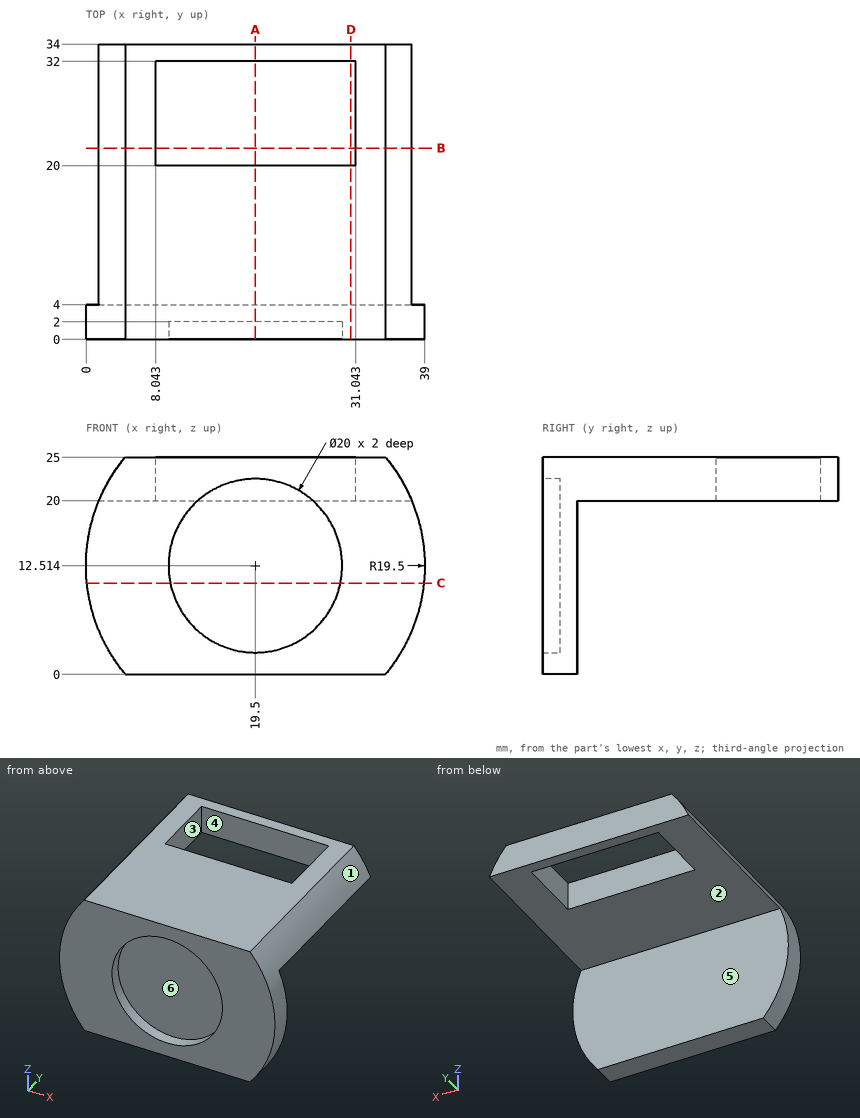
Could you check a few things on this drawing? It's one solid part, dimensions in mm from its lowest x, y, z. A direction names the side the tool comes from. Give positions to 0.01 mm unless a question says otherwise; leave off trailing zeros. Write each loop counter-clockwise with the first axis right and the second up, starting at its lowest first coordinate (ties: lowest second). Pieces come first, ordered by that corner, then holes. Notation, with made-up numbers: M 6.5,-5 L 64.5,-5 A14 cw 64.5,20 Z; hole C 31.5,9.5 d4. An arc over 180 degrees is marked long. Put each result on its own line as item: value. Start each with the question number.
Item 1: If we section it at C-C, the plane z = 10.5: Write out the boundary of the cut face in (x, y) (1 decimal), then the cut area to 3 significant figures.
Item 2: If we section it at B-B, the plane y = 22: Write out the boundary of the cut face in (x, z).
Item 3: Thinking about a two-plate mould opening in X: for the marked faces 1, 2 and 3, which applies, +X half, -X half, draft (parallel to the pull), parting line (faces both ways), or undercut?
Item 4: If we section it at D-D, the plane x = 30.5: Write out the boundary of the cut face in (y, z).
Item 5: I need wall thicknesses on L1, parallel to Y at x = 25.5, z = 22.5; L2, parallel to Z at x = 19.5, y = 1.3; L3, parallel to Y at x = 33, z = 6. Which ranges of each line are inside material? Lowest first, please. Write a range as from..to.
Item 6: On a 3-axis mill with a long thin cutter (end or side, diameter ignored), from which of +Z, -Z, +X, -X, +Y, -Y can I reach the whole of each face in a straight line? I mean the marked faces 4, 5 and 6. Say none if no direction works.
Item 7: If we section it at A-A, the plane x = 19.5: Write out the boundary of the cut face in (y, z).
Item 8: Will these pins go through, and if not, where does the flat tip stop? pin 1 (4 mm diameter, centred on y = 25, z = 21.5, fed in from +X); pin 2 (1.5 mm diameter, centred on y = 26, z = 21.5, fed in from -X) (1 decimal); pin 3 (1.5 mm diameter, centred on x = 30, y = 30, fed in from +Z); pin 4 (5 mm diameter, centred on x = 20, z = 19, fed in from -Y).
Values:
1. outline: M 0.1,0 L 9.7,0 L 9.7,2 L 29.3,2 L 29.3,0 L 38.9,0 L 38.9,4 L 0.1,4 Z
1. area: 116 mm²
2. outline: M 1.49,20 L 8.04,20 L 8.04,25 L 4.52,25 A19.5 ccw Z; M 31.04,20 L 37.51,20 A19.5 ccw 34.48,25 L 31.04,25 Z
3. face 1: +X half
3. face 2: draft
3. face 3: undercut
4. outline: M 0,0 L 4,0 L 4,20 L 20,20 L 20,25 L 0,25 Z; M 32,20 L 34,20 L 34,25 L 32,25 Z
5. L1: 0..20, 32..34
5. L2: 0..2.51, 22.51..25
5. L3: 0..4
6. face 4: +Z, -Z
6. face 5: -Z, +X, -X, +Y
6. face 6: -Y
7. outline: M 0,0 L 4,0 L 4,20 L 20,20 L 20,25 L 0,25 L 0,22.51 L 2,22.51 L 2,2.51 L 0,2.51 Z; M 32,20 L 34,20 L 34,25 L 32,25 Z
8. pin 1: x = 37.51
8. pin 2: x = 1.8
8. pin 3: through
8. pin 4: y = 2
